```python
from build123d import *

# Parameters (mm, degrees)
F0_R           = 55.1311075469
F2_DEPTH       = 25.4
F3_D           = 5.5
F3_CBORE_D     = 9.75
F3_CBORE_DEPTH = 5
F4_D           = 6.6
F4_CBORE_D     = 11.25
F4_CBORE_DEPTH = 6


with BuildPart() as f2:
    # F0 (on Front) → F2 (new body)
    with BuildSketch(Plane.XZ):
        Circle(F0_R)
    extrude(amount=F2_DEPTH)

    # F3 (through all)
    with Locations(Plane(origin=(0, 0, 0), x_dir=(1, 0, 0), z_dir=(0, 1, 0))):
        with Locations((-32.6479577467, -32.6479577467), (0, -46.1711846292), (32.6479577467, -32.6479577467), (46.1711846292, 0), (32.6479577467, 32.6479577467), (0, 46.1711846292), (-46.1711846292, 0), (-32.6479577467, 32.6479577467)):
            CounterBoreHole(F3_D / 2, F3_CBORE_D / 2, F3_CBORE_DEPTH)

    # F4 (through all)
    with Locations(Plane(origin=(0, 0, 0), x_dir=(1, 0, 0), z_dir=(0, 1, 0))):
        with Locations((-12.3326523611, 24.660010453), (0.9552987674, 26.0185740339), (-23.0103954673, -12.1819740161), (-15.1898693293, -23.0103954673), (22.0550966999, -13.8366000177), (27.5225216905, -1.6496149857)):
            CounterBoreHole(F4_D / 2, F4_CBORE_D / 2, F4_CBORE_DEPTH)


solid = f2.part
```
Geometry: final body of the model. Coordinates: model frame, mm. A direction names the side the tool comes from. Give positions to 0.01 mm unless a question says otherwise; leave off trailing zeros. Loops run counter-clockwise (first coordinate to the right, second up) from the corner with the lowest first, then second, coordinate; pieces in that order, holes last. Notation, with made-up numbers: (67, 42.25) -> (80, 42.25) arc R18 cw to (80, 67.25) -> close; hole circle Ø9 at (37.5, 31). An arc over 180 degrees is marked (long way). Use one line per item in the form item = value.
Item 1: Section query C-C on y = -2.5. Give the number of separate pieces and of enclosed holes in the cut face, and give its area (3 significant figures).
A:
separate_pieces = 1
enclosed_holes = 14
area = 8,350 mm^2
Item 2: Section query D-D on x = 11.5. Output: boundary loops of the cut face in (y, z).
A:
outline = (-25.4, -53.92) -> (0, -53.92) -> (0, 53.92) -> (-25.4, 53.92) -> close
Item 3: Access query for faces 1 (the face through (-13.55, -2.96, -19.17)), 2 (the face through (48.92, -15.34, -0.12)). Directions: +Z, -Z, +X, -X, +Y, -Y. A direction counts if a zero-diameter tool reaches every point of the face in a straight line with its end or side. Return the directions, or none.
A:
face_1 = +Y
face_2 = +Y, -Y
Item 4: Line query: probe 1 along X at (y, z) = (-3, 1); probe 2 along Z at (x, y) = (25, -13.25); probe 3 along Z at (x, y) = (0, -2.95). Output: solid intervals per line, ascending.
A:
probe_1 = -55.12 to -50.94, -41.4 to 21.94, 33.11 to 41.4, 50.94 to 55.12
probe_2 = -49.14 to -0.48, 3.78 to 12.35, 15.33 to 49.14
probe_3 = -55.13 to -51.05, -41.3 to -31.56, -20.48 to 41.3, 51.05 to 55.13
Item 5: Section query A-A on x = 0. Output: boundary loops of the cut face in (y, z).
A:
outline = (-25.4, -55.13) -> (0, -55.13) -> (0, -51.05) -> (-5, -51.05) -> (-5, -48.92) -> (-25.4, -48.92) -> close; (-25.4, -43.42) -> (-5, -43.42) -> (-5, -41.3) -> (0, -41.3) -> (0, -31.56) -> (-6, -31.56) -> (-6, -29.18) -> (-25.4, -29.18) -> close; (-25.4, -22.86) -> (-6, -22.86) -> (-6, -20.48) -> (0, -20.48) -> (0, 41.3) -> (-5, 41.3) -> (-5, 43.42) -> (-25.4, 43.42) -> close; (-25.4, 48.92) -> (-5, 48.92) -> (-5, 51.05) -> (0, 51.05) -> (0, 55.13) -> (-25.4, 55.13) -> close
Item 6: Draft query along X for faces 3 (the face through (-46.806, -2.465, -4.834)), 4 (the face through (-27.474, -2.958, 15.605)). Return one class per face: pulls with the +X half, pulls with the -X half, needs draft (parallel to the pull), parting line crosses it, or undercut.
A:
face_3 = undercut
face_4 = undercut
Item 7: Section query B-B on z = 0. Output: boundary loops of the cut face in (x, y), and give its area (3 significant figures).
A:
outline = (-55.13, -25.4) -> (-48.92, -25.4) -> (-48.92, -5) -> (-51.05, -5) -> (-51.05, 0) -> (-55.13, 0) -> close; (-43.42, -25.4) -> (24.66, -25.4) -> (24.66, -6) -> (22.14, -6) -> (22.14, 0) -> (-41.3, 0) -> (-41.3, -5) -> (-43.42, -5) -> close; (30.38, -25.4) -> (43.42, -25.4) -> (43.42, -5) -> (41.3, -5) -> (41.3, 0) -> (32.9, 0) -> (32.9, -6) -> (30.38, -6) -> close; (48.92, -25.4) -> (55.13, -25.4) -> (55.13, 0) -> (51.05, 0) -> (51.05, -5) -> (48.92, -5) -> close
area = 2,300 mm^2
Item 8: Pin query (flat end, axial travel): P1, Ø5, axis at x = -46.17, z = 0, coming from the +Y side; P2, Ø3, axis at x = 6.5, y = -4.5, coming from the +Z side; P3, Ø1.5, axis at x = -31, y = -19.5, coming from the +Z side; P4, Ø3, axis at x = -34.5, y = -9.5, coming from the +Z side. Return the tip coordinate at first contact, or that it passes through.
A:
P1 = through
P2 = 54.9
P3 = 46.09
P4 = 44.16
